```python
from build123d import *

# Parameters (mm, degrees)
F0_W      = 1860.55
F0_H      = 1403.35
F2_DEPTH  = 254
F3_W      = 1708.15
F3_H      = 50.8
F4_DEPTH  = 203.2
F5_W      = 101.6
F5_H      = 965.2
F5_H_2    = 196.85
F6_DEPTH  = 152.4
F7_W      = 508
F7_H      = 196.85
F8_DEPTH  = 203.2
F9_W      = 101.6
F9_H      = 965.2
F9_H_2    = 196.85
F10_DEPTH = 133.35


with BuildPart() as f2:
    # F0 (on Front) → F2 (new body)
    with BuildSketch(Plane.XZ):
        with Locations((930.275, 701.675)):
            Rectangle(F0_W, F0_H)
    extrude(amount=-F2_DEPTH)

    # F3 (on face) → F4 (join)
    with BuildSketch(Plane.XZ):
        with Locations((930.275, 1339.85)):
            Rectangle(F3_W, F3_H)
    extrude(amount=F4_DEPTH)

    # F5 (on face) → F6 (join)
    with BuildSketch(Plane.XZ):
        Polygon((152.4, 1314.45), (152.4, 0), (355.6, 0), (355.6, 1016), (1504.95, 1016), (1504.95, 0), (1708.15, 0), (1708.15, 1314.45), align=None)
        with Locations((254, 533.4)):
            Rectangle(F5_W, F5_H, mode=Mode.SUBTRACT)
        with Locations((1606.55, 533.4)):
            Rectangle(F5_W, F5_H, mode=Mode.SUBTRACT)
        with Locations((254, 1165.225)):
            Rectangle(F5_W, F5_H_2, mode=Mode.SUBTRACT)
        with Locations((1606.55, 1165.225)):
            Rectangle(F5_W, F5_H_2, mode=Mode.SUBTRACT)
    extrude(amount=F6_DEPTH)

    # F7 (on face) → F8 (cut)
    with BuildSketch(Plane.XZ.offset(152.4)):
        with Locations((930.275, 1165.225)):
            Rectangle(F7_W, F7_H)
    extrude(amount=-F8_DEPTH, mode=Mode.SUBTRACT)

    # F9 (on face) → F10 (join)
    with BuildSketch(Plane.XZ):
        with Locations((254, 533.4)):
            Rectangle(F9_W, F9_H)
        with Locations((254, 1165.225)):
            Rectangle(F9_W, F9_H_2)
        with Locations((1606.55, 1165.225)):
            Rectangle(F9_W, F9_H_2)
        with Locations((1606.55, 533.4)):
            Rectangle(F9_W, F9_H)
    extrude(amount=F10_DEPTH)


solid = f2.part
```
Here's how the part is built. I have some questions about the finished solid (model axes, mm). A direction names the side the tool comes from. Coordinates: 2 decimals unless noted, no trailing zeros. Loops run counter-clockwise (first coordinate to the right, second up) from the corner with the lowest first, then second, coordinate; pieces in that order, holes last. Notation, with made-up numbers: (24.25, -38.75) - (53.25, -38.75) arc R32 ccw to (53.25, -10.75) - close; hole circle Ø8 at (68, 87). An arc over 180 degrees is marked (long way). Answer as CSV lines item,"result".
Q1. For pin 1 (4 mm diameter, centred on x = 817.5, y = -59, fed in from +Z); pin 2 (9.5 mm diameter, centred on y = -138.5, z = 1124.5, fed in from +X); pin 3 (5.5 mm diameter, centred on x = 1597.5, y = -141.5, fed in from -Z); pin 4 (1.5 mm diameter, centred on x = 898.5, z = 1110, fed in from -Y), each with a flat end and sliding along its axis, tell me the tip position at first contact or that it passes through.
Response:
pin 1,"z = 1365.25"
pin 2,"x = 1708.15"
pin 3,"z = 0"
pin 4,"y = 50.8"
Q2. If we section it at C-C, the plane x = 1452: Write out the boundary of the cut face in (y, z), and give its area (3 significant figures).
Response:
outline,"(-203.2, 1314.45) - (-152.4, 1314.45) - (-152.4, 1016) - (0, 1016) - (0, 0) - (254, 0) - (254, 1403.35) - (0, 1403.35) - (0, 1365.25) - (-203.2, 1365.25) - close"
area,"412,000 mm2"
Q3. For faces 1 (the face through (927, -52, 1263.65)), 2 (the face through (76.2, -100, 1339)), 3 (the face through (918, -100, 1365.25)), 4 (the face through (355.6, -75, 501)), which set-ups out of +Z, -Z, +X, -X, +Y, -Y let a thin tool reach every point of the face, with its end or its side?
Response:
face 1,"-Y"
face 2,"+Z, -Z, -X, -Y"
face 3,"+Z, +X, -X, -Y"
face 4,"-Z, -Y"
Q4. If we section it at A-A, the plane x = 238.5: Write out the boundary of the cut face in (y, z).
Response:
outline,"(-203.2, 1314.45) - (-152.4, 1314.45) - (-152.4, 1263.65) - (-133.35, 1263.65) - (-133.35, 1066.8) - (-152.4, 1066.8) - (-152.4, 1016) - (-133.35, 1016) - (-133.35, 50.8) - (-152.4, 50.8) - (-152.4, 0) - (254, 0) - (254, 1403.35) - (0, 1403.35) - (0, 1365.25) - (-203.2, 1365.25) - close"
Q5. If I drill on L1, parallel to X at y = -16, z = 991.5; L2, parallel to X at y = -26.5, z = 1040.5; L3, parallel to Y at x = 1474.5, z = 387, over which ranges is the centre line in solid material (lowest first)? Write a range as [from, to].
Response:
L1,"[152.4, 355.6], [1504.95, 1708.15]"
L2,"[152.4, 1708.15]"
L3,"[0, 254]"
Q6. We'd pull the mould along X, two halves only. Please class faces 5 (the face through (927, 50.8, 1167)), 6 (the face through (1860.55, 125, 692)), 7 (the face through (253, -133.35, 540)), 8 (the face through (869, -152.4, 1050)): pulls with the +X half, pulls with the -X half, needs draft (parallel to the pull), parting line crosses it, or undercut.
Response:
face 5,"undercut"
face 6,"pulls with the +X half"
face 7,"undercut"
face 8,"needs draft"
Q7. If we section it at D-D, the plane z = 1162: Write out the boundary of the cut face in (x, y) (3 decimals), and give its area (3 significant figures).
Response:
outline,"(0, 0) - (152.4, 0) - (152.4, -152.4) - (203.2, -152.4) - (203.2, -133.35) - (304.8, -133.35) - (304.8, -152.4) - (676.275, -152.4) - (676.275, 50.8) - (1184.275, 50.8) - (1184.275, -152.4) - (1555.75, -152.4) - (1555.75, -133.35) - (1657.35, -133.35) - (1657.35, -152.4) - (1708.15, -152.4) - (1708.15, 0) - (1860.55, 0) - (1860.55, 254) - (0, 254) - close"
area,"603,000 mm2"
Q8. If we section it at B-B, the plane z = 167: Write out the boundary of the cut face in (x, y), and give its area (3 significant figures).
Response:
outline,"(0, 0) - (152.4, 0) - (152.4, -152.4) - (203.2, -152.4) - (203.2, -133.35) - (304.8, -133.35) - (304.8, -152.4) - (355.6, -152.4) - (355.6, 0) - (1504.95, 0) - (1504.95, -152.4) - (1555.75, -152.4) - (1555.75, -133.35) - (1657.35, -133.35) - (1657.35, -152.4) - (1708.15, -152.4) - (1708.15, 0) - (1860.55, 0) - (1860.55, 254) - (0, 254) - close"
area,"531,000 mm2"
